Answer from the drawing. Dimensions are ordinates in mm from the lowest x, y and z of the part. Coordinates: 2 decimals unless noted, no trailing zeros. Write each loop counter-clockwise with the first axis right and the second up, starting at its lowest first coordinate (ties: lowest second). Pieces come first, ordered by that corner, then holes. Notation, with made-up numbers: (64.5, 32) -> (111.5, 32) arc R34 ccw to (111.5, 69) -> close; hole circle Ø6 at (41, 29). An arc over 180 degrees is marked (long way). Answer as a JSON object with one key per item and string values. Group by question number.
(1) Find section C-C (y = 23.5). Give the vertices of the cut face in (x, z), then the cut area to 3 significant figures.
(2) Find section B-B (x = 13.5). Give the vertices of the cut face in (y, z).
(3) Find section A-A (z = 12.5). Give the vertices of the cut face in (x, y).
(4) Straight lines are drawn through the part: L1, parallel to Z at x = 79.5, y = 24.5; L2, parallel to X at y = 22.5, z = 18; L3, parallel to X at y = 12.5, z = 12. For each, find the intervals that lie inside material, in ascending order.
(5) A flat-ended cylindrical pin translates along its axis: P1, Ø5, axis at x = 79.5, z = 12.5, coming from the +Y side. Find the tip coordinate at first contact, or state that the pin passes through.
(6) For a pull along X with two mould halves and no side action, classify the marked faces 1, 2 and 3 as +X half, -X half, draft (parallel to the pull), parting line (faces both ways), or undercut.
(7) Find section D-D (z = 5.5). Give the vertices of the cut face in (x, y).
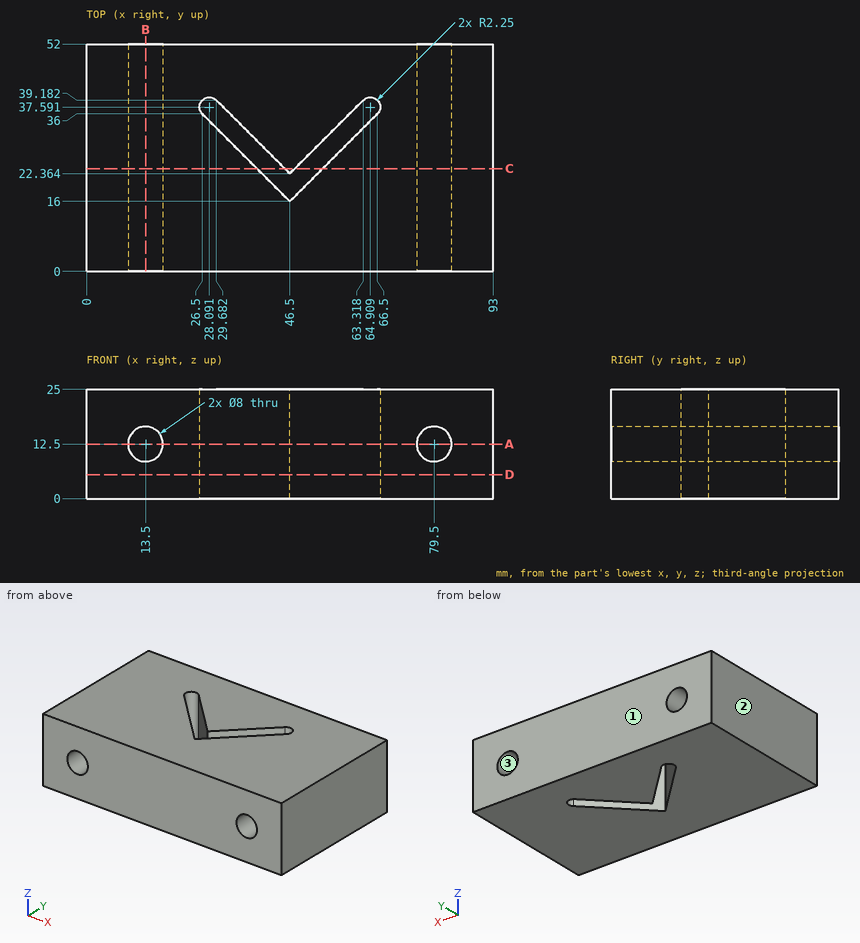
Results below:
{
 "1": {"outline": "(0, 0) -> (39, 0) -> (39, 25) -> (0, 25) -> close; (45.36, 0) -> (47.64, 0) -> (47.64, 25) -> (45.36, 25) -> close; (54, 0) -> (93, 0) -> (93, 25) -> (54, 25) -> close; hole circle Ø8 at (13.5, 12.5); hole circle Ø8 at (79.5, 12.5)", "area": "1,910 mm2"},
 "2": {"outline": "(0, 0) -> (52, 0) -> (52, 8.5) -> (0, 8.5) -> close; (0, 16.5) -> (52, 16.5) -> (52, 25) -> (0, 25) -> close"},
 "3": {"outline": "(0, 0) -> (9.5, 0) -> (9.5, 52) -> (0, 52) -> close; (17.5, 0) -> (75.5, 0) -> (75.5, 52) -> (17.5, 52) -> close; (83.5, 0) -> (93, 0) -> (93, 52) -> (83.5, 52) -> close; hole (26.5, 36) -> (46.5, 16) -> (66.5, 36) arc R2.25 ccw to (63.32, 39.18) -> (46.5, 22.36) -> (29.68, 39.18) arc R2.25 ccw to start"},
 "4": {"L1": "z = 0 to 8.5, 16.5 to 25", "L2": "x = 0 to 40, 46.36 to 46.64, 53 to 93", "L3": "x = 0 to 9.53, 17.47 to 75.53, 83.47 to 93"},
 "5": {"P1": "passes through"},
 "6": {"face 1": "draft", "face 2": "-X half", "face 3": "undercut"},
 "7": {"outline": "(0, 0) -> (93, 0) -> (93, 52) -> (0, 52) -> close; hole (26.5, 36) -> (46.5, 16) -> (66.5, 36) arc R2.25 ccw to (63.32, 39.18) -> (46.5, 22.36) -> (29.68, 39.18) arc R2.25 ccw to start"}
}
